Geometry check sheet. Reference: the model listing, model coordinates, mm. A direction names the side the tool comes from. Round coordinates to 2 decimals unless told otherwise and drop trailing zeros. Order: outer loops, then holes, each group sorted by start corner. A loop starts at its lowest first (then second) coordinate and runs counter-clockwise, first axis right, second up. Notation, with made-up numbers: (67.25, 29.25) - (125.25, 29.25) arc R31 ccw to (125.25, 66.25) - close; hole circle Ø10 at (35.25, -4.5). An arc over 180 degrees is marked (long way). Use a Markdown table: item, result. Add a question column.
(1) Section check A-A on z = 0. Record the boundary of the cut face in (x, y).
(2) Mould release check, pull along Z, two halves, no side actions. Record for faces 4 (the face through (3.3, 16.6, 55)), 5 (the face through (19, 150, -45)), 6 (the face through (14.418, 73.95, 45.783)): released by +Z, released by -Z, zero draft, split by the parting line, or undercut.
(3) Section check D-D on y = 59.5. Record the boundary of the cut face in (x, z), then the cut area to 3 significant figures.
(4) Section check B-B on x = 0. Record the boundary of the cut face in (y, z), then the cut area to 3 significant figures.
(5) Gauge pin test, flat ends, axial feed: P1, Ø1, axis at x = -28, y = 113.5, coming from the +Z side; P2, Ø12, axis at y = 16.5, z = -23, coming from the +X side; P3, Ø4, axis at x = 0, y = 18.79, coming from the +Z side; P4, Ø2, axis at y = 98.5, z = 7.5, coming from the +X side. Record the tip position at first contact, or that the pin passes through.
(6) Section check C-C on x = -33. Record the boundary of the cut face in (y, z).
(7) Thickness scan on line 1 along Z through (x, y) = (0, 119); line 2 along Y through (x, z) = (0, -52); line 3 along Z through (x, y) = (9, 29). Record the ranges inside material, lowest first. Write a range as [from, to].
(8) Access from +Z, -Z, +X, -X, +Y, -Y to the whole of each face (thin tool, end or side, straight path). Record for faces 1 (the face through (19, 0, -45)), 2 (the face through (-1.08, 13.91, 52.41)), 3 (the face through (-1.08, 13.91, -52.41)).
```python
from build123d import *

# Parameters (mm, degrees)
SKETCH1_R                = 50
SKETCH1_R_2              = 48
BOSS_EXTRUDE2_DEPTH      = 150
BOSS_EXTRUDE3_REACH      = 191.803
BOSS_EXTRUDE3_END_RADIUS = 50
SKETCH2_R                = 5
SKETCH3_R                = 3.5
CUT_EXTRUDE1_DEPTH       = 12
BOSS_EXTRUDE4_REACH      = 194.614
BOSS_EXTRUDE4_END_RADIUS = 50
SKETCH4_R                = 5
CUT_EXTRUDE2_START       = -12
SKETCH5_R                = 3.5
CUT_EXTRUDE2_DEPTH       = 12


with BuildPart() as part:
    # Sketch1 → Boss-Extrude2 (new body)
    with BuildSketch(Plane(origin=(0, 0, 0), x_dir=(1, 0, 0), z_dir=(0, 1, 0))):
        with Locations(Location((0, 0, 0), (0, 0, 270))):
            Circle(SKETCH1_R)
        with Locations(Location((0, 0, 0), (0, 0, 270))):
            Circle(SKETCH1_R_2, mode=Mode.SUBTRACT)
    extrude(amount=BOSS_EXTRUDE2_DEPTH)

    # Boss-Extrude3: up to this cylinder (the profile starts outside it)
    boss_extrude3_end = Plane(origin=(0, 18.790559, 0), z_dir=(0, -1, 0)) * Cylinder(BOSS_EXTRUDE3_END_RADIUS, 484.606, mode=Mode.PRIVATE)
    # Sketch2 → Boss-Extrude3 (add, up to the surface)
    with BuildSketch(Plane.XY.offset(55), mode=Mode.PRIVATE) as boss_extrude3_sk1:
        with Locations((0, 18.790558937)):
            Circle(SKETCH2_R)
    boss_extrude3_tool1 = extrude(boss_extrude3_sk1.sketch, amount=-BOSS_EXTRUDE3_REACH, mode=Mode.PRIVATE) - boss_extrude3_end
    add(boss_extrude3_tool1.solids().sort_by_distance((0, 18.790559, 55))[0])

    # Sketch3 → Cut-Extrude1 (cut)
    with BuildSketch(Plane.XY.offset(55)):
        with Locations((0, 18.790558937)):
            Circle(SKETCH3_R)
    extrude(amount=-CUT_EXTRUDE1_DEPTH, mode=Mode.SUBTRACT)

    # Boss-Extrude4: up to this cylinder (the profile starts outside it)
    boss_extrude4_end = Plane(origin=(0, 18.790559, 0), z_dir=(0, -1, 0)) * Cylinder(BOSS_EXTRUDE4_END_RADIUS, 490.228, mode=Mode.PRIVATE)
    # Sketch4 → Boss-Extrude4 (add, up to the surface)
    with BuildSketch(Plane.XY.offset(-55), mode=Mode.PRIVATE) as boss_extrude4_sk1:
        with Locations((0, 18.790558937)):
            Circle(SKETCH4_R)
    boss_extrude4_tool1 = extrude(boss_extrude4_sk1.sketch, amount=BOSS_EXTRUDE4_REACH, mode=Mode.PRIVATE) - boss_extrude4_end
    add(boss_extrude4_tool1.solids().sort_by_distance((0, 18.790559, -55))[0])

    # Sketch5 → Cut-Extrude2 (cut)
    with BuildSketch(Plane(origin=(0, 0, -55), x_dir=(-1, 0, 0), z_dir=(0, 0, -1)).offset(CUT_EXTRUDE2_START)):
        with Locations(Location((0, 18.790558937, 0), (0, 0, 180))):
            Circle(SKETCH5_R)
    extrude(amount=CUT_EXTRUDE2_DEPTH, mode=Mode.SUBTRACT)


solid = part.part
```
Check sheet entries:
| question | item | result |
|---|---|---|
| 1 | outline | (-50, 0) - (-48, 0) - (-48, 150) - (-50, 150) - close; (48, 0) - (50, 0) - (50, 150) - (48, 150) - close |
| 2 | face 4 | released by +Z |
| 2 | face 5 | zero draft |
| 2 | face 6 | undercut |
| 3 | outline | circle Ø100 at (0, 0); hole circle Ø96 at (0, 0) |
| 3 | area | 616 mm2 |
| 4 | outline | (0, -50) - (13.79, -50) - (13.79, -55) - (15.29, -55) - (15.29, -48) - (0, -48) - close; (0, 48) - (15.29, 48) - (15.29, 55) - (13.79, 55) - (13.79, 50) - (0, 50) - close; (22.29, -55) - (23.79, -55) - (23.79, -50) - (150, -50) - (150, -48) - (22.29, -48) - close; (22.29, 48) - (150, 48) - (150, 50) - (23.79, 50) - (23.79, 55) - (22.29, 55) - close |
| 4 | area | 602 mm2 |
| 5 | P1 | stops at z = 41.76 |
| 5 | P2 | stops at x = 47.02 |
| 5 | P3 | passes through |
| 5 | P4 | stops at x = 49.58 |
| 6 | outline | (0, -37.56) - (150, -37.56) - (150, -34.86) - (0, -34.86) - close; (0, 34.86) - (150, 34.86) - (150, 37.56) - (0, 37.56) - close |
| 7 | line 1 | z = [-50, -48], [48, 50] |
| 7 | line 2 | y = [13.79, 15.29], [22.29, 23.79] |
| 7 | line 3 | z = [-49.18, -47.15], [47.15, 49.18] |
| 8 | face 1 | +Z, -Z, +X, -X, -Y |
| 8 | face 2 | +Z |
| 8 | face 3 | -Z |
